```python
from build123d import *

# Parameters (mm, degrees)
F1_DEPTH  = 40
F2_DEPTH  = 2
F3_DEPTH  = 2
F4_W      = 25.2149685806
F4_H      = 2
F5_DEPTH  = 42.1
F5_FACE_W = 40.9870653462
F5_FACE_H = 2
F7_W      = 25.2149685806
F7_H      = 2
F8_DEPTH  = 42
F8_FACE_W = 40.9870653462
F8_FACE_H = 2
F10_W     = 21.6691600519
F10_H     = 33.2297814414
F11_DEPTH = 5.3


with BuildPart() as f1:
    # F0 (on Top) → F1 (new body)
    with BuildSketch(Plane.XY):
        Polygon((-13.4906232357, 20.567771814), (-24.4906232357, 20.567771814), (-39.384083382, 20.567771814), (-61.3453843386, -2.2496986568), (-39.33704599, -23.432228186), (-13.4906232357, -23.432228186), (-13.530928939, -21.9322283479), (-38.732458267, -21.9322283479), (-59.2244518674, -2.2091464562), (-38.7458975196, 19.0677719759), (-24.530928939, 19.0677719759), (-13.530928939, 19.0677719759), align=None)
    extrude(amount=F1_DEPTH)

    # F2 (add): a face of the model
    f2_faces = [f1.faces().sort_by_distance(p)[0] for p in [
        (-49.4292616832, -12.5390688822, 40),
    ]]
    extrude(f2_faces, amount=F2_DEPTH)

    # F3 (add): a face of the model
    f3_faces = [f1.faces().sort_by_distance(p)[0] for p in [
        (-49.4292616832, -12.5390688822, 42),
    ]]
    extrude(f3_faces, amount=F3_DEPTH)

    # F4 (on face) → F5 (join)
    with BuildSketch(Plane.XZ.offset(-19.0677719759)):
        with Locations((-26.1384132293, 43)):
            Rectangle(F4_W, F4_H)
    extrude(amount=F5_DEPTH)

    # F5_face (on face) → F6 (join, up to the next surface of F1)
    with BuildSketch(Plane(origin=(-38.7458975196, -1.4257606972, 43), x_dir=(0, -1, 0), z_dir=(-1, 0, 0))):
        Rectangle(F5_FACE_W, F5_FACE_H)
    extrude(until=Until.NEXT)

    # F7 (on face) → F8 (join)
    with BuildSketch(Plane.XZ.offset(-19.0677719759)):
        with Locations((-26.1384132293, 1)):
            Rectangle(F7_W, F7_H)
    extrude(amount=F8_DEPTH)

    # F8_face (on face) → F9 (join, up to the next surface of F1)
    with BuildSketch(Plane(origin=(-38.7458975196, -1.4257606972, 1), x_dir=(0, -1, 0), z_dir=(-1, 0, 0))):
        Rectangle(F8_FACE_W, F8_FACE_H)
    extrude(until=Until.NEXT)

    # F10 (on face) → F11 (cut)
    with BuildSketch(Plane(origin=(-30.7211592709, 29.5684232548, 0), x_dir=(-0.6934601651, -0.7204949684, 0), z_dir=(-0.7204949684, 0.6934601651, 0))):
        with Locations((28.3268968852, 22.3851092793)):
            Rectangle(F10_W, F10_H)
    extrude(amount=-F11_DEPTH, mode=Mode.SUBTRACT)


solid = f1.part
```
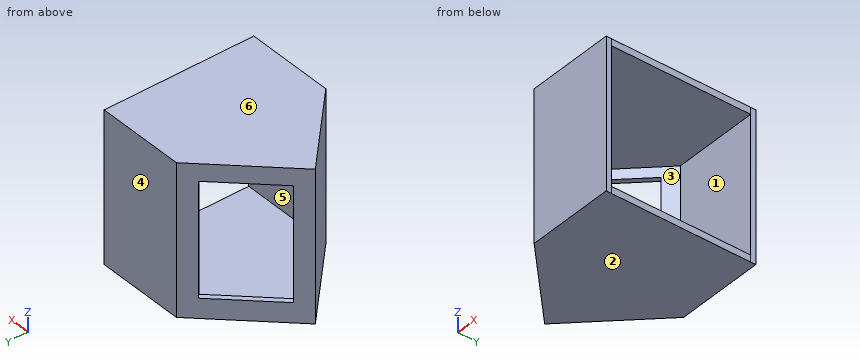
Source: CAD feature listing. Evaluate the final solid. Frame: model axes, mm. Face numbers are marked on the shaded views. A direction names the side the tool comes from. Coordinates: 2 decimals unless noted, no trailing zeros. Loops run counter-clockwise (first coordinate to the right, second up) from the corner with the lowest first, then second, coordinate; pieces in that order, holes last. Notation, with made-up numbers: (16, 14.5) -> (24, 14.5) arc R18 ccw to (24, 38.5) -> close; hole circle Ø10 at (15.5, 85.25). An arc over 180 degrees is marked (long way). One line per item, written item: value. Start each with the question number.
Q1. Line query: line 1 along Z through (x, y) = (-43, -13); line 2 along Y through (x, z) = (-23.5, 29); line 3 along Z through (x, y) = (-53, 5.5). Output: solid intervals per line, ascending.
Q2. Section query A-A, the plane z = 15. Return the cut outline in (x, y), and give its area (3 significant figures).
Q3. Section query C-C, the plane y = 4.5. Return the cut outline in (x, z), and give its area (3 significant figures).
Q4. Section query B-B, the plane x = -23. Return the cut outline in (y, z), and give its area (3 significant figures).
Q5. Mould query, pull axis Z, two halves, no side actions, for the marked faces 3, 4, 5 and 6. Classes: pulls with the +Z half, pulls with the -Z half, needs draft (parallel to the pull), parting line crosses it, or undercut.
Q6. Section query D-D, the plane z = 5. Return the cut outline in (x, y).
Q7. Set-up query: the marked faces 1 and 2. Return all of +Z, -Z, +X, -X, +Y, -Y with unobstructed straight access to the full face (end or side cutting, diameter ignored); none if empty.
Q8. Contact query for flat-ended pins moving along their axis: P1, Ø8, axis at x = -49, z = 30.5, coming from the +Y side; P2, Ø0.6, axis at y = 3, z = 43, coming from the +X side; P3, Ø1, axis at x = -46, z = 38, coming from the +Y side. Output: stop coordinate, or through.
Results:
1. line 1: 0 to 2, 42 to 44
1. line 2: -23.43 to -21.93, 19.07 to 20.57
1. line 3: 0 to 5.77, 39 to 44
2. outline: (-61.35, -2.25) -> (-39.34, -23.43) -> (-13.49, -23.43) -> (-13.53, -21.93) -> (-38.73, -21.93) -> (-59.22, -2.21) -> (-56.8, 0.31) -> (-57.88, 1.35) -> close; (-42.85, 16.97) -> (-41.77, 15.93) -> (-38.75, 19.07) -> (-13.53, 19.07) -> (-13.49, 20.57) -> (-39.38, 20.57) -> close
2. area: 134 mm^2
3. outline: (-54.85, 0) -> (-13.53, 0) -> (-13.53, 2) -> (-52.77, 2) -> (-52.77, 5.77) -> (-54.85, 5.77) -> close; (-54.85, 39) -> (-52.77, 39) -> (-52.77, 42) -> (-13.53, 42) -> (-13.53, 44) -> (-54.85, 44) -> close
3. area: 179 mm^2
4. outline: (-23.43, 0) -> (20.57, 0) -> (20.57, 44) -> (-23.43, 44) -> close; hole (-21.93, 2) -> (19.07, 2) -> (19.07, 42) -> (-21.93, 42) -> close
4. area: 296 mm^2
5. face 3: undercut
5. face 4: needs draft
5. face 5: undercut
5. face 6: pulls with the +Z half
6. outline: (-61.35, -2.25) -> (-39.34, -23.43) -> (-13.49, -23.43) -> (-13.53, -21.93) -> (-38.73, -21.93) -> (-59.22, -2.21) -> (-38.75, 19.07) -> (-13.53, 19.07) -> (-13.49, 20.57) -> (-39.38, 20.57) -> close
7. face 1: +X
7. face 2: -Z, +X, -X, +Y, -Y
8. P1: y = -8.2
8. P2: x = -13.53
8. P3: y = -14.46
